The model under review builds one solid part; all positions refer to its coordinate system, in mm. Coordinates: 2 decimals unless noted, no trailing zeros. Loops run counter-clockwise (first coordinate to the right, second up) from the corner with the lowest first, then second, coordinate; pieces in that order, holes last. Notation, with made-up numbers: M 17,45.25 L 63,45.25 A27 ccw 63,65.25 Z; hole C -33.75,59 d9. An arc over 180 degrees is marked long. One line per item, written item: value.
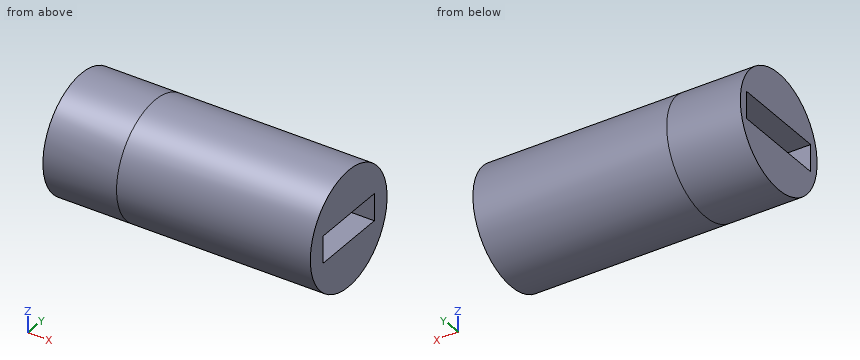
```python
from build123d import *

# Parameters (mm, degrees)
SKETCH1_R           = 3
SKETCH1_W           = 1.4
SKETCH1_H           = 4
BOSS_EXTRUDE1_DEPTH = 10
BOSS_EXTRUDE2_START = 3.8
SKETCH2_R           = 3
SKETCH2_W           = 1.4
SKETCH2_H           = 5
BOSS_EXTRUDE2_DEPTH = 3.8


with BuildPart() as part:
    # Sketch1 → Boss-Extrude1 (new body)
    with BuildSketch(Plane(origin=(0, 0, 0), x_dir=(0, 0, -1), z_dir=(1, 0, 0))):
        Circle(SKETCH1_R)
        Rectangle(SKETCH1_W, SKETCH1_H, mode=Mode.SUBTRACT)
    extrude(amount=BOSS_EXTRUDE1_DEPTH)

    # Sketch2 → Boss-Extrude2 (add)
    with BuildSketch(Plane.ZY.offset(BOSS_EXTRUDE2_START)):
        Circle(SKETCH2_R)
        Rectangle(SKETCH2_W, SKETCH2_H, mode=Mode.SUBTRACT)
    extrude(amount=-BOSS_EXTRUDE2_DEPTH)


solid = part.part
```
(1) Add section A-A on z = 0. State the section outline as (x, y) points.
Checks:
outline: M -3.8,-3 L 10,-3 L 10,-2 L 0,-2 L 0,-2.5 L -3.8,-2.5 Z; M -3.8,2.5 L 0,2.5 L 0,2 L 10,2 L 10,3 L -3.8,3 Z
(2) To check wall thickness, follow L1, parallel to X at y = -2.4, z = 0.15; L2, parallel to Z at x = 6.5, y = -0.45; L3, parallel to Z at x = -2.5, y = 0.6. State the ranges of each line that lie inside material, in increasing order. Write a range as [from, to].
Checks:
L1: [0, 10]
L2: [-2.97, -0.7], [0.7, 2.97]
L3: [-2.94, -0.7], [0.7, 2.94]
(3) Add section C-C on x = 5.25. State the section outline as (y, z) points, then the cut area to 3 significant figures.
Checks:
outline: C 0,0 d6; hole M -2,-0.7 L 2,-0.7 L 2,0.7 L -2,0.7 Z
area: 22.7 mm^2
(4) Add section B-B on y = 0. State the section outline as (x, z) points.
Checks:
outline: M -3.8,-3 L 10,-3 L 10,-0.7 L -3.8,-0.7 Z; M -3.8,0.7 L 10,0.7 L 10,3 L -3.8,3 Z
(5) Insertion check: pin 1 Ø1 at (x, y) = (0.5, 2) entering from -Z. The pin has a flat end and moves straight along its axis. Give the tip position at first contact, or say it passes through.
Checks:
pin 1: z = -2.6
(6) Add section D-D on x = -2. State the section outline as (y, z) points, then the cut area to 3 significant figures.
Checks:
outline: C 0,0 d6; hole M -2.5,-0.7 L 2.5,-0.7 L 2.5,0.7 L -2.5,0.7 Z
area: 21.3 mm^2
